The figure shows three views and two pictorial views of one solid part (mm, origin at its lowest corner). Answer the questions. A direction names the side the tool comes from. Coordinates: 2 decimals unless noted, no trailing zeros. Loops run counter-clockwise (first coordinate to the right, second up) from the corner with the lowest first, then second, coordinate; pieces in that order, holes last.
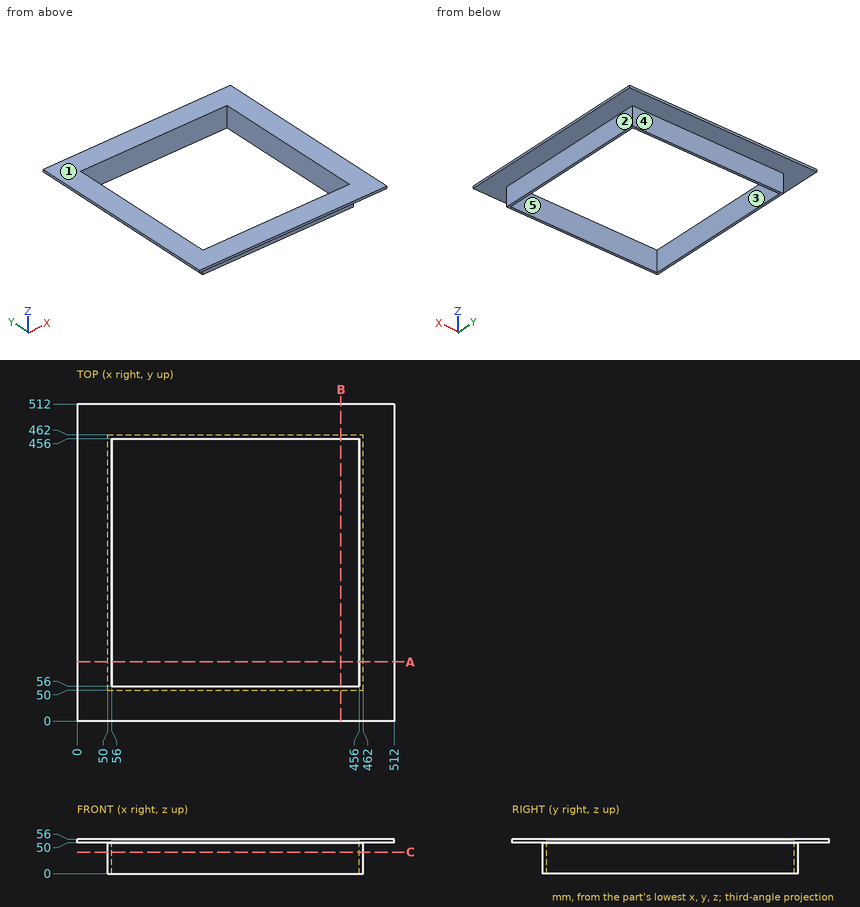
1. Straight lines are drawn through the part: probe 1 along X at (y, z) = (156.5, 49); probe 2 along Y at (x, z) = (283, 52). For each, find the intervals that lie inside material, in ascending order.
2. Determine the mould class of the marked faces 1, 2 and 3 for opening direction X: released by +X, released by -X, zero draft, split by the parting line, or undercut.
3. Each of these flat-tipped pins is pushed along its axis until it touches: P1, Ø8, axis at x = 343, z = 20.5, coming from the -Y side; P2, Ø1.5, axis at y = 345, z = 19, coming from the -X side; P3, Ø25, axis at x = 223, z = 36, coming from the +Y side. Where does it stop, or does it pass through?
4. A cutting plane is placed at C-C, the plane z = 35. Give the vertices of the cut face in (x, y).
5. A cutting plane is placed at A-A, the plane y = 95.5. Give the vertices of the cut face in (x, z), then the cut area to 3 significant figures.
6. For the marked faces 4 and 5, determine the directions among +Z, -Z, +X, -X, +Y, -Y from which every point of the face is accessible in a straight line to the end or side of a thin tool.
Answers below:
1. probe 1: x = 50 to 56, 456 to 462
1. probe 2: y = 0 to 56, 456 to 512
2. face 1: zero draft
2. face 2: released by +X
2. face 3: undercut
3. P1: stops at y = 50
3. P2: stops at x = 50
3. P3: stops at y = 462
4. outline: (50, 50) - (462, 50) - (462, 462) - (50, 462) - close; hole (56, 56) - (456, 56) - (456, 456) - (56, 456) - close
5. outline: (0, 50) - (50, 50) - (50, 0) - (56, 0) - (56, 56) - (0, 56) - close; (456, 0) - (462, 0) - (462, 50) - (512, 50) - (512, 56) - (456, 56) - close
5. area: 1,270 mm2
6. face 4: -Z, +X, -X, +Y
6. face 5: +Z, -Z
